from build123d import *

# Parameters (mm, degrees)
BOSS_EXTRUDE1_DEPTH = 38.1
CUT_EXTRUDE2_DEPTH  = 76.2
FILLET1_R           = 6.35
SKETCH10_W          = 21.59
SKETCH10_H          = 76.2
CUT_EXTRUDE3_DEPTH  = 76.2
FILLET2_R           = 2.54
FILLET3_R           = 2.54
SKETCH11_R          = 6.5024
CUT_EXTRUDE4_DEPTH  = 76.2
SKETCH12_R          = 6.35
CUT_EXTRUDE5_DEPTH  = 76.2


with BuildPart() as part:
    # Sketch7 → Boss-Extrude1 (new, symmetric)
    with BuildSketch(Plane.XY):
        Polygon((0, 0), (0, 63.5), (3.81, 63.5), (3.81, 3.81), (63.5, 3.81), (63.5, 0), align=None)
    extrude(amount=BOSS_EXTRUDE1_DEPTH, both=True)

    # Sketch8 → Cut-Extrude2 (cut)
    with BuildSketch(Plane(origin=(3.81, 0, 0), x_dir=(0, 0, -1), z_dir=(1, 0, 0))):
        Polygon((-38.1, 63.5), (-38.1, 3.81), (0, 63.5), align=None)
        Polygon((38.1, 63.5), (0, 63.5), (38.1, 3.81), align=None)
    extrude(amount=-CUT_EXTRUDE2_DEPTH, mode=Mode.SUBTRACT)

    # Fillet1
    fillet1_edges = [part.edges().sort_by_distance(p)[0] for p in [
        (1.905, 63.5, 0),
    ]]
    fillet(fillet1_edges, radius=FILLET1_R)

    # Sketch10 → Cut-Extrude3 (cut)
    with BuildSketch(Plane(origin=(0, 3.81, 0), x_dir=(1, 0, 0), z_dir=(0, 1, 0))):
        with Locations((52.705, 0)):
            Rectangle(SKETCH10_W, SKETCH10_H)
    extrude(amount=-CUT_EXTRUDE3_DEPTH, mode=Mode.SUBTRACT)

    # Fillet2
    fillet2_edges = [part.edges().sort_by_distance(p)[0] for p in [
        (0, 1.905, 38.1),
        (0, 1.905, -38.1),
        (41.91, 1.905, -38.1),
        (41.91, 1.905, 38.1),
    ]]
    fillet(fillet2_edges, radius=FILLET2_R)

    # Fillet3
    fillet3_edges = [part.edges().sort_by_distance(p)[0] for p in [
        (3.81, 3.81, 0),
    ]]
    fillet(fillet3_edges, radius=FILLET3_R)

    # Sketch11 → Cut-Extrude4 (cut)
    with BuildSketch(Plane(origin=(3.81, 0, 0), x_dir=(0, 0, -1), z_dir=(1, 0, 0))):
        with Locations((0, 42.692021475)):
            Circle(SKETCH11_R)
    extrude(amount=-CUT_EXTRUDE4_DEPTH, mode=Mode.SUBTRACT)

    # Sketch12 → Cut-Extrude5 (cut)
    with BuildSketch(Plane(origin=(0, 3.81, 0), x_dir=(1, 0, 0), z_dir=(0, 1, 0))):
        with Locations(Location((22.86, 19.05, 0), (0, 0, 180))):
            Circle(SKETCH12_R)
        with Locations(Location((22.86, -19.05, 0), (0, 0, 180))):
            Circle(SKETCH12_R)
    extrude(amount=-CUT_EXTRUDE5_DEPTH, mode=Mode.SUBTRACT)


solid = part.part
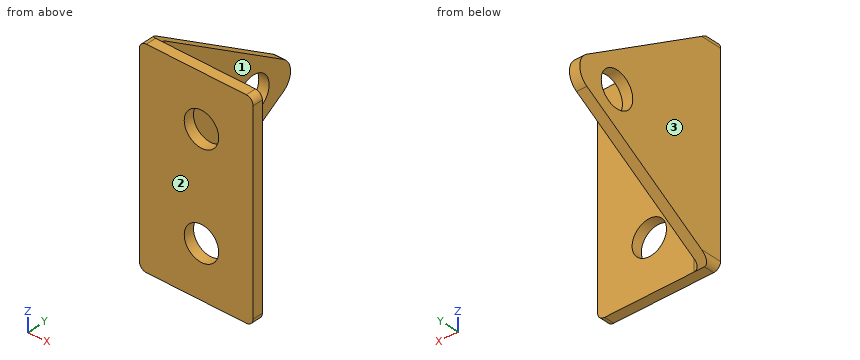
Here's how the part is built. I have some questions about the finished solid (model axes, mm). Face numbers are marked on the shaded views. Give positions to 0.01 mm unless a question says otherwise; leave off trailing zeros. Order: outer loops, then holes, each group sorted by start corner. A loop starts at its lowest first (then second) coordinate and runs counter-clockwise, first axis right, second up. Notation, with made-up numbers: M 17.25,11 L 25.25,11 A24 cw 25.25,46 Z; hole C 25,8.25 d9. An arc over 180 degrees is marked long. Answer as a JSON object with one key per item and string values. Group by question number.
1) Please list where these lines run through material, in increasing order: L1, parallel to X at y = 1, z = -19; L2, parallel to Y at x = 24, z = 28.5. Write a range as [from, to].
2) Suppose I cut it at B-B, the plane x = 22. Write out the boundary of the cut face in (y, z), plus the area to 3 significant figures.
3) Suppose I cut it at D-D, the plane z = 33. Write out the boundary of the cut face in (x, y).
4) I'm going to push flat-ended pins straight in: pin 1 Ø8 at (y, z) = (42.69, 0) entering from +X; pin 2 Ø10 at (y, z) = (22, -9.5) entering from +X; pin 3 Ø20.5 at (x, z) = (22.86, 19.05) entering from +Y. Where does each tip first touch, or does it pass through?
5) Suppose I cut it at C-C, the plane y = 38.5. Write out the boundary of the cut face in (x, z).
6) We'd pull the mould along X, two halves only. Please class the marked faces 1, 2 and 3: pulls with the +X half, pulls with the -X half, needs draft (parallel to the pull), parting line crosses it, or undercut.
7) Suppose I cut it at A-A, the plane z = 0. Write out the boundary of the cut face in (x, y), plus the area to 3 significant figures.
Results found:
{
 "1": {"L1": "[0, 16.51], [29.21, 41.91]", "L2": "[0, 3.81]"},
 "2": {"outline": "M 0,-38.1 L 3.81,-38.1 L 3.81,-25.34 L 0,-25.34 Z; M 0,-12.76 L 3.81,-12.76 L 3.81,12.76 L 0,12.76 Z; M 0,25.34 L 3.81,25.34 L 3.81,38.1 L 0,38.1 Z", "area": "194 mm²"},
 "3": {"outline": "M 0,0 L 41.91,0 L 41.91,3.81 L 6.35,3.81 A2.54 cw 3.81,6.35 L 3.81,11.8 L 0,11.8 Z"},
 "4": {"pin 1": "through", "pin 2": "x = 3.81", "pin 3": "y = 3.81"},
 "5": {"outline": "M 0,-15.96 L 3.81,-15.96 L 3.81,-4.97 L 0,-4.97 Z; M 0,4.97 L 3.81,4.97 L 3.81,15.96 L 0,15.96 Z"},
 "6": {"face 1": "pulls with the +X half", "face 2": "needs draft", "face 3": "pulls with the -X half"},
 "7": {"outline": "M 0,0 L 41.91,0 L 41.91,3.81 L 6.35,3.81 A2.54 cw 3.81,6.35 L 3.81,36.19 L 0,36.19 Z; M 0,49.19 L 3.81,49.19 L 3.81,58.05 L 0,58.05 Z", "area": "318 mm²"}
}
